Read the model definition and answer for the solid it produces. Units are mm, in the model's axes. A direction names the side the tool comes from. Coordinates: 2 decimals unless noted, no trailing zeros. Loops run counter-clockwise (first coordinate to the right, second up) from the corner with the lowest first, then second, coordinate; pieces in that order, holes last. Notation, with made-up numbers: (29, 60) - (73, 60) arc R19 ccw to (73, 97) - close; hole circle Ø1 at (23.5, 55). An arc over 180 degrees is marked (long way). Use one line per item in the form item = value. Start each with the question number.
1) A cutting plane is placed at B-B (y = 6.75). Give the vertices of the cut face in (x, z), and give its area (3 significant figures).
2) The mould has two halves that part along X. Classify faces 5 (the face through (-2, 5, -6)), 6 (the face through (10.59, 0.54, 10.47)), 7 (the face through (9.861, 0.006, 8.103)), 8 (the face through (-8.75, -6, 6)): released by +X, released by -X, zero draft, split by the parting line, or undercut.
3) A cutting plane is placed at C-C (z = 19.5). Give the vertices of the cut face in (x, y), and give its area (3 significant figures).
4) Which of the six approach directions +Z, -Z, +X, -X, +Y, -Y give full straight-line access (tool end or side, diameter ignored) to faces 1 (the face through (-2, 2.75, -3)), 2 (the face through (-8.75, 6, 6)), 3 (the face through (8.75, 6, 6)), 4 (the face through (-2, 7.75, -3))?
5) A cutting plane is placed at A-A (x = 0). Give the vertices of the cut face in (y, z), and give its area (3 significant figures).
6) Consider line 1 (X direction, y = 0, z = 9.5); line 2 (Y direction, x = 10, z = 9.95); line 3 (X direction, y = 5.75, z = 12). Determine where each line is inside the solid, lowest interval first.
7) A cutting plane is placed at D-D (z = 14.5). Give the vertices of the cut face in (x, y), and give its area (3 significant figures).
8) Each of these flat-tipped pins is pushed along its axis until it touches: P1, Ø1.9, axis at y = 5, z = 7.5, coming from the +X side; P2, Ø1.9, axis at y = -7, z = 4, coming from the -X side; P3, Ø6.5, axis at x = -3.5, z = -3.5, coming from the -Y side. Where does it stop, or does it pass through?
from build123d import *

# Parameters (mm, degrees)
F0_W     = 17.5
F0_H     = 17.5
F1_DEPTH = 12.5
F2_R     = 7.75
F3_DEPTH = 15
F5_DEPTH = 12.5
F6_D     = 1.6
F6_DEPTH = 4
F6_TIP   = 0.4806884952
F7_W     = 5.7
F7_H     = 5
F8_DEPTH = 6
F9_W     = 2.6
F9_H     = 5.5


with BuildPart() as f1:
    # F0 (on Top) → F1 (new body)
    with BuildSketch(Plane.XY):
        Rectangle(F0_W, F0_H)
    extrude(amount=F1_DEPTH)

    # F2 (on face) → F3 (join)
    with BuildSketch(Plane.XY.offset(12.5)):
        Circle(F2_R)
    extrude(amount=F3_DEPTH)

    # F4 (on face) → F5 (join, through all)
    with BuildSketch(Plane.XY.offset(12.5)):
        with BuildLine():
            Line((10, 2.5), (-10, 2.5))
            ThreePointArc((-10, 2.5), (-12.5, 0), (-10, -2.5))
            Line((-10, -2.5), (10, -2.5))
            ThreePointArc((10, -2.5), (12.5, 0), (10, 2.5))
        make_face()
    extrude(amount=-F5_DEPTH)

    # F6
    with Locations(Plane.XY.offset(12.5)):
        with Locations((-10, 0), (10, 0)):
            Hole(F6_D / 2, depth=F6_DEPTH)
            with Locations((0, 0, -(F6_DEPTH + F6_TIP / 2))):  # 118° drill point
                Cone(0, F6_D / 2, F6_TIP, mode=Mode.SUBTRACT)

    # F7 (on Top) → F8 (join)
    with BuildSketch(Plane.XY):
        with Locations((-2.35, 5.25)):
            Rectangle(F7_W, F7_H)
    extrude(amount=-F8_DEPTH)

    # F9 (on face) → F10 (join, up to the next surface of F1)
    with BuildSketch(Plane(origin=(0, 8.75, 0), x_dir=(-1, 0, 0), z_dir=(0, 1, 0))):
        with Locations((0, 15.25)):
            Rectangle(F9_W, F9_H)
    extrude(until=Until.NEXT, dir=(0, -1, 0))


solid = f1.part
Found:
q1.outline = (-8.75, 0) - (-5.2, 0) - (-5.2, -6) - (0.5, -6) - (0.5, 0) - (8.75, 0) - (8.75, 12.5) - (3.81, 12.5) - (3.81, 27.5) - (-3.81, 27.5) - (-3.81, 12.5) - (-8.75, 12.5) - close
q1.area = 367 mm^2
q2.face_5 = zero draft
q2.face_6 = undercut
q2.face_7 = undercut
q2.face_8 = released by -X
q3.outline = circle Ø15.5 at (0, 0)
q3.area = 189 mm^2
q4.face_1 = -Z, +X, -X, -Y
q4.face_2 = +Z, -Z, -X, +Y
q4.face_3 = +Z, -Z, +X, +Y
q4.face_4 = -Z, +X, -X, +Y
q5.outline = (-8.75, 0) - (2.75, 0) - (2.75, -6) - (7.75, -6) - (7.75, 0) - (8.75, 0) - (8.75, 18) - (7.75, 18) - (7.75, 27.5) - (-7.75, 27.5) - (-7.75, 12.5) - (-8.75, 12.5) - close
q5.area = 487 mm^2
q6.line_1 = -12.5 to -10.8, -9.2 to 9.2, 10.8 to 12.5
q6.line_2 = -2.5 to -0.8, 0.8 to 2.5
q6.line_3 = -8.75 to 8.75
q7.outline = (-1.3, 7.64) arc R7.75 ccw (long way) to (1.3, 7.64) - (1.3, 8.75) - (-1.3, 8.75) - close
q7.area = 191 mm^2
q8.P1 = 8.75
q8.P2 = -8.75
q8.P3 = 2.75
